Check sheet for the modelled part. Datum: model origin and axes. Units: mm. Face numbers are marked on the shaded views. A direction names the side the tool comes from. Give positions to 0.01 mm unless a question says otherwise; leave off trailing zeros. Order: outer loops, then holes, each group sorted by start corner. A loop starts at its lowest first (then second) coordinate and runs counter-clockwise, first axis right, second up. Notation, with made-up numbers: (11.5, 33) - (30.5, 33) arc R12 cw to (30.5, 50) - close; hole circle Ø6 at (36, 14.5). An arc over 180 degrees is marked (long way). Answer in a Markdown table with one row per item.
from build123d import *

# Parameters (mm, degrees)
SKETCH1_W                 = 30
SKETCH1_H                 = 9.5
CUT_EXTRUDE1_DEPTH        = 3.5
SKETCH3_R                 = 17.4
BOSS_EXTRUDE1_DEPTH       = 4
SKETCH4_R                 = 10
BOSS_EXTRUDE2_DEPTH       = 16
CUT_EXTRUDE2_DEPTH        = 50.759421218
SKETCH6_W                 = 4
SKETCH6_H                 = 26
M4X0_7_TAPPED_HOLE1_D     = 3.3
M3X0_5_TAPPED_HOLE1_D     = 2.5
M3X0_5_TAPPED_HOLE1_DEPTH = 7.5
M3X0_5_TAPPED_HOLE1_TIP   = 0.751075774
FILLET1_R                 = 2
SKETCH15_W                = 1.25
SKETCH15_H                = 30


with BuildPart() as part:
    # Sketch1 → Revolve1 (revolve)
    with BuildSketch(Plane.XZ, mode=Mode.PRIVATE) as revolve1_sk:
        with Locations((15, 5.25)):
            Rectangle(SKETCH1_W, SKETCH1_H)
    revolve(revolve1_sk.sketch.rotate(Axis((0, 0, 10), (0, 0, -1)), 180), axis=Axis((0, 0, 10), (0, 0, -1)))

    # Sketch2 → Cut-Extrude1 (cut)
    with BuildSketch(Plane(origin=(0, 0, 0.5), x_dir=(-1, 0, 0), z_dir=(0, 0, -1))):
        with BuildLine():
            ThreePointArc((-14.379253383, 22.852506912), (-27, 0), (-14.379253383, -22.852506912))
            ThreePointArc((-14.379253383, -22.852506912), (-13.103370267, -25.060195635), (-10.562335147, -24.848281153))
            ThreePointArc((-10.562335147, -24.848281153), (-6.318658968, -26.250229501), (-1.901854596, -26.932934283))
            ThreePointArc((-1.901854596, -26.932934283), (0, -27.88125), (1.901854596, -26.932934283))
            ThreePointArc((1.901854596, -26.932934283), (6.318658968, -26.250229501), (10.562335147, -24.848281153))
            ThreePointArc((10.562335147, -24.848281153), (13.103370267, -25.060195635), (14.379253383, -22.852506912))
            ThreePointArc((14.379253383, -22.852506912), (27, 0), (14.379253383, 22.852506912))
            ThreePointArc((14.379253383, 22.852506912), (13.103370267, 25.060195635), (10.562335147, 24.848281153))
            ThreePointArc((10.562335147, 24.848281153), (6.318658968, 26.250229501), (1.901854596, 26.932934283))
            ThreePointArc((1.901854596, 26.932934283), (0, 27.88125), (-1.901854596, 26.932934283))
            ThreePointArc((-1.901854596, 26.932934283), (-6.318658968, 26.250229501), (-10.562335147, 24.848281153))
            ThreePointArc((-10.562335147, 24.848281153), (-13.103370267, 25.060195635), (-14.379253383, 22.852506912))
        make_face()
    extrude(amount=-CUT_EXTRUDE1_DEPTH, mode=Mode.SUBTRACT)

    # Sketch3 → Boss-Extrude1 (add)
    with BuildSketch(Plane(origin=(0, 0, 4), x_dir=(-1, 0, 0), z_dir=(0, 0, -1))):
        Circle(SKETCH3_R)
    extrude(amount=BOSS_EXTRUDE1_DEPTH)

    # Sketch4 → Boss-Extrude2 (add)
    with BuildSketch(Plane(origin=(0, 0, 0), x_dir=(-1, 0, 0), z_dir=(0, 0, -1))):
        Circle(SKETCH4_R)
    extrude(amount=BOSS_EXTRUDE2_DEPTH)

    # Sketch5 → Cut-Extrude2 (cut, through all)
    with BuildSketch(Plane.XY.offset(10)):
        with BuildLine():
            Line((-1, 5), (-1, 3.872983346))
            ThreePointArc((-1, 3.872983346), (0, 4), (1, 3.872983346))
            Line((1, 3.872983346), (1, 5))
            Line((1, 5), (-1, 5))
        make_face()
    extrude(amount=-CUT_EXTRUDE2_DEPTH, mode=Mode.SUBTRACT)

    # Sketch6 → Cut-Revolve1 (revolve, cut)
    with BuildSketch(Plane.XZ):
        with Locations((2, -3)):
            Rectangle(SKETCH6_W, SKETCH6_H)
    revolve(axis=Axis((0, 0, 10), (0, 0, -1)), mode=Mode.SUBTRACT)

    # M4x0.7 Tapped Hole1 (through all)
    with Locations(Plane.XY.offset(10)):
        with Locations((-12, -22.95), (0, -25.5), (12, -22.95), (12, 22.95), (0, 25.5), (-12, 22.95)):
            Hole(M4X0_7_TAPPED_HOLE1_D / 2)

    # M3x0.5 Tapped Hole1
    with Locations(Plane(origin=(0, 0, -16), x_dir=(-1, 0, 0), z_dir=(0, 0, -1))):
        with Locations((-5.055813485, -5.055813485), (5.055813485, -5.055813485), (5.055813485, 5.055813485), (-5.055813485, 5.055813485)):
            Hole(M3X0_5_TAPPED_HOLE1_D / 2, depth=M3X0_5_TAPPED_HOLE1_DEPTH)
            with Locations((0, 0, -(M3X0_5_TAPPED_HOLE1_DEPTH + M3X0_5_TAPPED_HOLE1_TIP / 2))):  # 118° drill point
                Cone(0, M3X0_5_TAPPED_HOLE1_D / 2, M3X0_5_TAPPED_HOLE1_TIP, mode=Mode.SUBTRACT)

    # Fillet1
    fillet1_edges = [part.edges().sort_by_distance(p)[0] for p in [
        (10, 0, 0),
    ]]
    fillet(fillet1_edges, radius=FILLET1_R)

    # Sketch15 → M3x0.5 Tapped Hole2 (revolve, cut)
    with BuildSketch(Plane(origin=(0, 0, -8), x_dir=(0, 0, -1), z_dir=(1, 0, 0))):
        with Locations((0.625, 15)):
            Rectangle(SKETCH15_W, SKETCH15_H)
    revolve(axis=Axis((0, -6.35, -8), (0, 1, 0)), mode=Mode.SUBTRACT)


solid = part.part
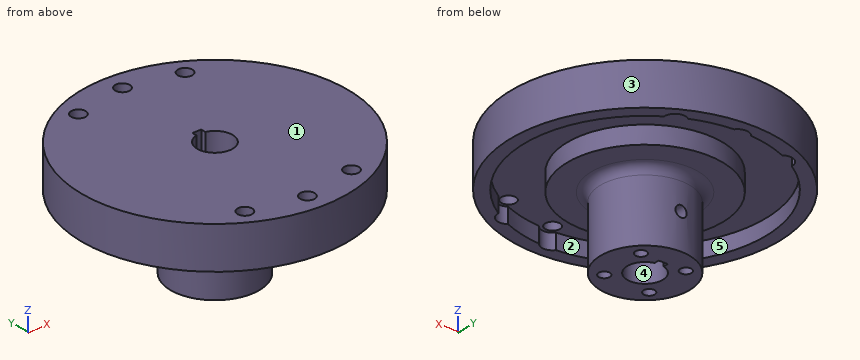
(1) Thickness scan on L1, parallel to Y at x = -12, z = 5.2; L2, parallel to X at y = 11.5, z = 0.75; L3, parallel to X at y = -21.5, z = 5.5. Record the ranges inside material, lowest first.
Geometry says:
| item | result |
|---|---|
| L1 | -27.5 to -24.6, -21.3 to 21.3, 24.6 to 27.5 |
| L2 | -27.71 to -24.43, -13.06 to 13.06, 24.43 to 27.71 |
| L3 | -20.92 to -12.79, -11.21 to 11.21, 12.79 to 20.92 |
(2) Cross-section at B-B, the plane y = 0. Record the cut outline in (x, z), then the cut area to 3 significant figures.
Geometry says:
| item | result |
|---|---|
| outline | (-30, 0.5) - (-27, 0.5) - (-27, 4) - (-17.4, 4) - (-17.4, 0) - (-12, 0) arc R2 cw to (-10, -2) - (-10, -16) - (-4, -16) - (-4, 10) - (-30, 10) - close; (4, -16) - (10, -16) - (10, -2) arc R2 cw to (12, 0) - (17.4, 0) - (17.4, 4) - (27, 4) - (27, 0.5) - (30, 0.5) - (30, 10) - (4, 10) - close |
| area | 634 mm² |
(3) Gauge pin test, flat ends, axial feed: P1, Ø10, axis at y = -21, z = 0, coming from the +X side; P2, Ø2, axis at x = 0, z = -8, coming from the +Y side; P3, Ø1, axis at x = -9, z = -6.5, coming from the -Y side. Record the tip position at first contact, or that the pin passes through.
Geometry says:
| item | result |
|---|---|
| P1 | x = 25.36 |
| P2 | y = -3.87 |
| P3 | y = -5.27 |
(4) Cross-section at A-A, the plane x = 0. Give the number of separate pieces and of enclosed holes in the cut face, then the cut area to 3 significant figures.
Geometry says:
| item | result |
|---|---|
| separate pieces | 5 |
| enclosed holes | 0 |
| area | 550 mm² |
(5) Access from +Z, -Z, +X, -X, +Y, -Y to the whole of each face (thin tool, end or side, straight path). Record for the marked faces 4 and 5.
Geometry says:
| item | result |
|---|---|
| face 4 | +Z, -Z |
| face 5 | -Z |
(6) Mould release check, pull along X, two halves, no side actions. Record for the marked faces 1, 2 and 3: pulls with the +X half, pulls with the -X half, needs draft (parallel to the pull), parting line crosses it, or undercut.
Geometry says:
| item | result |
|---|---|
| face 1 | needs draft |
| face 2 | undercut |
| face 3 | parting line crosses it |
(7) Cross-section at D-D, the plane z = -0.75. Record the cut outline in (x, y), then the cut area to 3 significant figures.
Geometry says:
| item | result |
|---|---|
| outline | circle Ø20.88 at (0, 0); hole (-1, 3.87) arc R4 ccw (long way) to (1, 3.87) - (1, 5) - (-1, 5) - close |
| area | 290 mm² |
(8) Cross-section at C-C, the plane x = 21.5. Record the cut outline in (y, z).
Geometry says:
| item | result |
|---|---|
| outline | (-20.92, 0.5) - (-16.33, 0.5) - (-16.33, 4) - (16.33, 4) - (16.33, 0.5) - (20.92, 0.5) - (20.92, 10) - (-20.92, 10) - close |
